The model under review builds one solid part; all positions refer to its coordinate system, in mm. Give positions to 0.01 mm unless a question says otherwise; leave off trailing zeros. Loops run counter-clockwise (first coordinate to the right, second up) from the corner with the lowest first, then second, coordinate; pieces in that order, holes last. Notation, with made-up numbers: (-34.75, -0.75) - (-21.75, -0.75) arc R27 ccw to (-21.75, 20.25) - close; hole circle Ø7 at (-24, 1.25). An arc over 180 degrees is marked (long way). Return JSON: item names as keys, results as strings. Group by question number.
from build123d import *

# Parameters (mm, degrees)
F0_R     = 1.560353
F1_DEPTH = 10


with BuildPart() as f1:
    # F0 (on Front) → F1 (new body)
    with BuildSketch(Plane.XZ):
        with BuildLine():
            ThreePointArc((-4.160941, 24.608993), (-4.032911, 21.89542), (-4.160941, 19.181847))
            Line((-4.160941, 19.181847), (-4.160941, -29.993249))
            Line((-4.160941, -29.993249), (-2.5, -45.391009))
            Line((-2.5, -45.391009), (2.5, -45.391009))
            Line((2.5, -45.391009), (4.161059, -29.993249))
            Line((4.161059, -29.993249), (4.161059, 15.619488))
            Line((4.161059, 15.619488), (4.160941, 19.181847))
            ThreePointArc((4.160941, 19.181847), (4.032911, 21.89542), (4.160941, 24.608993))
            ThreePointArc((4.160941, 24.608993), (0, 28.769934), (-4.160941, 24.608993))
        make_face()
        with Locations((0, 24.608993)):
            Circle(F0_R, mode=Mode.SUBTRACT)
    extrude(amount=F1_DEPTH)


solid = f1.part
Item 1: Mouldability with a two-part tool opening along X and no side actions: class faces 1 (the face through (-3.342, -4.93, -37.584)), 2 (the face through (0, -5, -45.391)), 3 (the face through (4.033, -4.93, 21.857)), 4 (the face through (-0.338, -4.93, 23.086)) as +X half, -X half, draft (parallel to the pull), parting line (faces both ways), or undercut.
Item 2: For L1, parallel to Z at x = 0, y = -3.25; L2, parallel to Z at x = 0.5, y = -4.5; L3, parallel to X at y = -6, z = 25, list the stretches that pass through material, from the lowest coordinate up. Write a range as from..to.
Item 3: Take a section at C-C (z = -37). State the section outline as (x, y) points.
Item 4: Take a section at A-A (x = 0). State the section outline as (y, z) points.
Item 5: Take a section at B-B (y = -7). State the section outline as (x, z) points.
Check sheet entries:
{
 "1": {"face 1": "-X half", "face 2": "draft", "face 3": "+X half", "face 4": "undercut"},
 "2": {"L1": "z = -45.39..23.05, 26.17..28.77", "L2": "z = -45.39..23.13, 26.09..28.74", "L3": "x = -4.14..-1.51, 1.51..4.14"},
 "3": {"outline": "(-3.41, -10) - (3.41, -10) - (3.41, 0) - (-3.41, 0) - close"},
 "4": {"outline": "(-10, -45.39) - (0, -45.39) - (0, 23.05) - (-10, 23.05) - close; (-10, 26.17) - (0, 26.17) - (0, 28.77) - (-10, 28.77) - close"},
 "5": {"outline": "(-4.16, -29.99) - (-2.5, -45.39) - (2.5, -45.39) - (4.16, -29.99) - (4.16, 15.62) - (4.16, 19.18) arc R28.82 cw to (4.16, 24.61) arc R4.16 ccw to (-4.16, 24.61) arc R28.82 cw to (-4.16, 19.18) - close; hole circle Ø3.12 at (0, 24.61)"}
}
